Build history of the part. All positions in model axes, mm. A direction names the side the tool comes from. Give positions to 0.01 mm unless a question says otherwise; leave off trailing zeros. Loops run counter-clockwise (first coordinate to the right, second up) from the corner with the lowest first, then second, coordinate; pieces in that order, holes last. Notation, with made-up numbers: M 9.5,60 L 68.5,60 A27 cw 68.5,86 Z; hole C 33.5,64 d4. An arc over 180 degrees is marked long. Answer as a JSON object with one key per item and string values. Group by question number.
1. Drill centre lines: line 1 along Z through (x, y) = (0, 6.5); line 2 along Z through (x, y) = (0, 4.35); line 3 along X through (y, z) = (5.6, 15.5). Where is each one in solid material? Low to high. Write a range as [from, to].
2. Slice it at B-B (x = 0). Give the number of separate pieces and of enclosed holes in the cut face, then the cut area to 3 significant figures.
3. Mould opens along X. For faces 1 (the face through (-25.855, 1.014, 17.407)), 2 (the face through (-25, 2, 17)), 3 (the face through (-16, 7.3, -16)) say: released by +X, released by -X, zero draft, split by the parting line, or undercut.
4. Slice it at A-A (z = 0). List the corners of the cut face in (x, y).
5. 3-axis set-ups, long thin cutter, end or side, ignore diameter. For faces 4 (the face through (8.767, 6.307, 16.856)), 5 (the face through (-23.03, 4.43, 14.3)), 6 (the face through (13, 5.3, -15)): which of +Z, -Z, +X, -X, +Y, -Y reach the whole face in a straight line?
6. Slice it at C-C (y = 3.5). List the corners of the cut face in (x, z).
7. Drop flat-ended pins along their axis: pin 1 Ø2.5 at (x, z) = (28.5, 15.5) entering from +Y; pin 2 Ø3 at (y, z) = (5, -27.5) entering from -X; pin 3 Ø4 at (x, z) = (-2, -32) entering from +Y. Give the stop position or say it passes through.
Autodesk Inventor part; units mm, degrees
ref_plane "YZ Plane" through (0, 0, 0) normal (1, 0, 0) x (0, 1, 0)
ref_plane "XZ Plane" through (0, 0, 0) normal (0, 1, 0) x (-1, 0, 0)
ref_plane "XY Plane" through (0, 0, 0) normal (0, 0, 1) x (1, 0, 0)
sketch "スケッチ1" plane through (0, 0, 0) normal (0, 1, 0) x (-1, 0, 0)
  circle A0 centre (0, 0) radius 37
  dimension "d0" = 74
extrude "押し出し1" add sketch "スケッチ1" along normal blind 7.3
sketch "スケッチ2" plane through (0, 7.3, 0) normal (0, 1, 0) x (1, 0, 0)
  circle A0 centre (0, 0) radius 19
  dimension "d3" = 38
extrude "押し出し2" cut sketch "スケッチ2" against normal through all
sketch "スケッチ3" plane through (0, 0, 0) normal (0, -1, 0) x (1, 0, 0)
  circle A0 centre (0, 0) radius 25.15
  dimension "d6" = 50.3
extrude "押し出し3" cut sketch "スケッチ3" against normal blind 5.3
sketch "スケッチ6" plane through (0, 7.3, 0) normal (0, 1, 0) x (1, 0, 0)
  circle A0 centre (0, 31) radius 2.15
  circle A1 centre (-26.8468, -15.5) radius 2.15
  circle A2 centre (26.8468, -15.5) radius 2.15
  point P0 (0, 0)
  dimension "d21" = 4.3
  dimension "d22" = 31
  dimension "d25" = 360
extrude "押し出し6" cut sketch "スケッチ6" against normal through all
sketch "スケッチ7" plane through (0, 7.3, 0) normal (0, 1, 0) x (1, 0, 0)
  circle A0 centre (0, 31) radius 2.15
  circle A1 centre (0, 31) radius 4
  circle A2 centre (-26.8468, -15.5) radius 4
  circle A3 centre (26.8468, -15.5) radius 4
  point P0 (0, 0)
  dimension "d29" = 8
  dimension "d32" = 360
extrude "押し出し7" cut sketch "スケッチ7" against normal blind 5.3 contours A0 | A1 | A2 | A3
chamfer "面取り1" distance 0.5 angle 45 8 edges at (37, 7.3, 0) (37, 0, 0) (-25.15, 0, 0) (-19, 7.3, 0) (-19, 5.3, 0) (22.8468, 7.3, 15.5) (-30.8468, 7.3, 15.5) (-4, 7.3, -31)
properties part number "clamp_for_bearing" material "ステンレス鋼"
Established:
{
 "1": {"line 1": "z = [-37, -35], [-27, -19], [19, 37]", "line 2": "z = [-37, -35], [-27, -25.15], [25.15, 37]", "line 3": "x = [-33.6, -30.85], [-22.85, -11.33], [11.33, 22.85], [30.85, 33.6]"},
 "2": {"separate pieces": "3", "enclosed holes": "0", "area": "145 mm^2"},
 "3": {"face 1": "undercut", "face 2": "undercut", "face 3": "zero draft"},
 "4": {"outline": "M -37,0.5 L -36.5,0 L -25.65,0 L -25.15,0.5 L -25.15,5.3 L -19.5,5.3 L -19,5.8 L -19,6.8 L -19.5,7.3 L -36.5,7.3 L -37,6.8 Z; M 19,5.8 L 19.5,5.3 L 25.15,5.3 L 25.15,0.5 L 25.65,0 L 36.5,0 L 37,0.5 L 37,6.8 L 36.5,7.3 L 19.5,7.3 L 19,6.8 Z"},
 "5": {"face 4": "+Y, -Y", "face 5": "+Y", "face 6": "-Y"},
 "6": {"outline": "C 0,0 d74; hole C -26.85,15.5 d8; hole C 0,0 d50.3; hole C 0,-31 d8; hole C 26.85,15.5 d8"},
 "7": {"pin 1": "stops at y = 2", "pin 2": "stops at x = -26.32", "pin 3": "stops at y = 7.04"}
}
